```python
from build123d import *

# Parameters (mm, degrees)
EXTRUDE_1_DEPTH     = 2.5
SKETCH_2_R          = 1.250000000000001
SKETCH_2_R_2        = 1.2499999999999991
CUT_EXTRUDE_1_DEPTH = 10
FILLET_1_R          = 1


with BuildPart() as part:
    # ｽｹｯﾁ1 → ﾎﾞｽ - 押し出し1 (new, symmetric)
    with BuildSketch(Plane(origin=(0, 0, 0), x_dir=(1, 0, 0), z_dir=(0, 1, 0))):
        with BuildLine():
            Line((-9.040153483210384, 4.275000000000001), (-17.500000000000004, 4.275000000000001))
            Line((-17.500000000000004, 4.275000000000001), (-17.5, -4.2749999999999995))
            Line((-17.5, -4.2749999999999995), (-9.040153483210384, -4.2749999999999995))
            ThreePointArc((-9.040153483210364, -4.2749999999999355), (-9.999999999999996, 2.09e-15), (-9.040153483210364, 4.27499999999994))
        make_face()
        with BuildLine():
            Line((-6.162335190493877, 4.275), (-9.040153483210384, 4.275000000000001))
            ThreePointArc((-9.040153483210364, 4.27499999999994), (-9.999999999999996, 2.09e-15), (-9.040153483210364, -4.2749999999999355))
            Line((-9.040153483210384, -4.2749999999999995), (-6.162335190493877, -4.2749999999999995))
            ThreePointArc((-6.162335190493898, -4.275000000000058), (-7.499999999999997, 1.79e-15), (-6.1623351904938986, 4.275000000000059))
        make_face()
        with BuildLine():
            ThreePointArc((10.000000000000004, 8.7e-16), (9.757088060279663, 2.1907150850688284), (9.040153483210378, 4.2749999999999195))
            Line((9.040153483210407, 4.2749999999999995), (6.162335190493945, 4.275))
            ThreePointArc((6.162335190493945, 4.275000000000002), (7.15777597891638, 2.2396970856898766), (7.500000000000004, 8.7e-16))
            ThreePointArc((7.500000000000004, -9.7e-16), (7.157775978916378, -2.2396970856898806), (6.162335190493939, -4.275000000000008))
            Line((6.162335190493941, -4.275), (9.04015348321041, -4.275))
            ThreePointArc((9.04015348321038, -4.274999999999914), (9.757088060279663, -2.190715085068826), (10.000000000000004, -1.58e-15))
        make_face()
        with BuildLine():
            ThreePointArc((9.040153483210378, 4.2749999999999195), (1.296e-14, 10), (-9.040153483210364, 4.27499999999994))
            Line((-9.040153483210384, 4.275000000000001), (-6.162335190493877, 4.275))
            ThreePointArc((-6.1623351904938986, 4.275000000000059), (3.724e-14, 7.500000000000002), (6.162335190493945, 4.275000000000002))
            Line((6.162335190493945, 4.275), (9.040153483210407, 4.2749999999999995))
        make_face()
        with BuildLine():
            Line((17.499999999999996, 4.2749999999999995), (9.040153483210407, 4.2749999999999995))
            ThreePointArc((9.040153483210378, 4.2749999999999195), (9.757088060279663, 2.1907150850688284), (10.000000000000004, 8.7e-16))
            ThreePointArc((10.000000000000004, -1.58e-15), (9.757088060279663, -2.190715085068826), (9.04015348321038, -4.274999999999914))
            Line((9.04015348321041, -4.275), (17.5, -4.275))
            Line((17.5, -4.275000000000001), (17.499999999999996, 4.2749999999999995))
        make_face()
        with BuildLine():
            Line((-6.162335190493877, -4.2749999999999995), (-9.040153483210384, -4.2749999999999995))
            ThreePointArc((-9.040153483210364, -4.2749999999999355), (1.94e-14, -10), (9.04015348321038, -4.274999999999914))
            Line((9.04015348321041, -4.275), (6.162335190493941, -4.275))
            ThreePointArc((6.162335190493939, -4.275000000000008), (3.54e-14, -7.5), (-6.162335190493898, -4.275000000000058))
        make_face()
    extrude(amount=EXTRUDE_1_DEPTH, both=True)

    # ｽｹｯﾁ2 → ｶｯﾄ - 押し出し1 (cut)
    with BuildSketch(Plane(origin=(2.1e-16, 0, -4.275), x_dir=(-1, 0, -5e-17), z_dir=(5e-17, 0, -1))):
        with Locations((14, 0)):
            Circle(SKETCH_2_R)
        with Locations((-14, 0)):
            Circle(SKETCH_2_R_2)
    extrude(amount=-CUT_EXTRUDE_1_DEPTH, mode=Mode.SUBTRACT)

    # ﾌｨﾚｯﾄ1
    fillet_1_edges = [part.edges().sort_by_distance(p)[0] for p in [
        (-9.040153483210375, 0, 4.274999999999968),
        (-9.040153483210375, 0, -4.27499999999997),
        (9.040153483210393, 0, -4.2749999999999595),
        (9.040153483210396, 0, 4.274999999999958),
    ]]
    fillet(fillet_1_edges, radius=FILLET_1_R)


solid = part.part
```
Can you work these out from the model? Positions are in its coordinate system, mm. A direction names the side the tool comes from. Give positions to 0.01 mm unless a question says otherwise; leave off trailing zeros. Order: outer loops, then holes, each group sorted by start corner. A loop starts at its lowest first (then second) coordinate and runs counter-clockwise, first axis right, second up. Notation, with made-up numbers: M -8.75,74 L -1.75,74 A18 cw -1.75,100 Z; hole C -12,67 d11. An arc over 180 degrees is marked long. Write item = value, one per line. Start each with the question number.
Q1. For faces 4 (the flat face through (12.6, 0, 4.275)), 5 (the flat face through (-13, -1, -4.275)), 6 (the flat face through (-13, 1, 4.275)), which set-ups out of +Z, -Z, +X, -X, +Y, -Y let a thin tool reach every point of the face, with its end or its side?
Q2. Suppose I cut it at C-C (y = 0). Write out the boundary of the cut face in (x, z) (3 decimals).
Q3. Will these pins go through, and if not, where does the flat tip stop? pin 1 Ø1.5 at (x, y) = (-13.5, -1) entering from +Z (3 decimals); pin 2 Ø3 at (y, z) = (1.5, 6) entering from -X; pin 3 Ø2.5 at (x, y) = (15, 0) entering from -Z (3 decimals).
Q4. Suppose I cut it at D-D (x = -14). Write out the boundary of the cut face in (y, z) (3 decimals).
Q5. Suppose I cut it at A-A (z = 0). Write out the boundary of the cut face in (x, y), plus the area to 3 significant figures.
Q6. Suppose I cut it at B-B (x = 0). Write out the boundary of the cut face in (y, z).
Q7. I need wall thicknesses on probe 1 along X at (y, z) = (0.2, 0); probe 2 along Y at (x, z) = (14, -2); probe 3 along X at (y, z) = (-0.7, 0). Which ranges of each line are inside material? Lowest first, please. Write a range as [from, to].
Q8. We'd pull the mould along Y, two halves only. Please class faces 1 (the cylindrical face through (-9.15, 0.04, 4.41)), 2 (the cylindrical face through (15.25, 0.05, -0.06)), 3 (the flat face through (8, -2.5, 0)): pulls with the +Y half, pulls with the -Y half, needs draft (parallel to the pull), parting line crosses it, or undercut.
Check result:
q1.face_4 = +Z, +X, +Y, -Y
q1.face_5 = -Z, -X, +Y, -Y
q1.face_6 = +Z, -X, +Y, -Y
q2.outline = M -17.5,-4.275 L -15.25,-4.275 L -15.25,4.275 L -17.5,4.275 Z; M -12.75,-4.275 L -9.653,-4.275 A1 cw -8.775,-4.795 A10 ccw 8.775,-4.795 A1 cw 9.653,-4.275 L 12.75,-4.275 L 12.75,4.275 L 9.653,4.275 A1 cw 8.775,4.795 A10 ccw -8.775,4.795 A1 cw -9.653,4.275 L -12.75,4.275 Z; M 15.25,-4.275 L 17.5,-4.275 L 17.5,4.275 L 15.25,4.275 Z; hole C 0,0 d15
q3.pin_1 = 4.275
q3.pin_2 = -9.02
q3.pin_3 = -4.275
q4.outline = M -2.5,-4.275 L -1.25,-4.275 L -1.25,4.275 L -2.5,4.275 Z; M 1.25,-4.275 L 2.5,-4.275 L 2.5,4.275 L 1.25,4.275 Z
q5.outline = M -17.5,-2.5 L -7.5,-2.5 L -7.5,2.5 L -17.5,2.5 Z; M 7.5,-2.5 L 17.5,-2.5 L 17.5,2.5 L 7.5,2.5 Z; hole C -14,0 d2.5; hole C 14,0 d2.5
q5.area = 90.2 mm2
q6.outline = M -2.5,-10 L 2.5,-10 L 2.5,-7.5 L -2.5,-7.5 Z; M -2.5,7.5 L 2.5,7.5 L 2.5,10 L -2.5,10 Z
q7.probe_1 = [-17.5, -15.23], [-12.77, -7.5], [7.5, 12.77], [15.23, 17.5]
q7.probe_2 = [-2.5, -1.25], [1.25, 2.5]
q7.probe_3 = [-17.5, -15.04], [-12.96, -7.5], [7.5, 12.96], [15.04, 17.5]
q8.face_1 = needs draft
q8.face_2 = undercut
q8.face_3 = pulls with the -Y half
